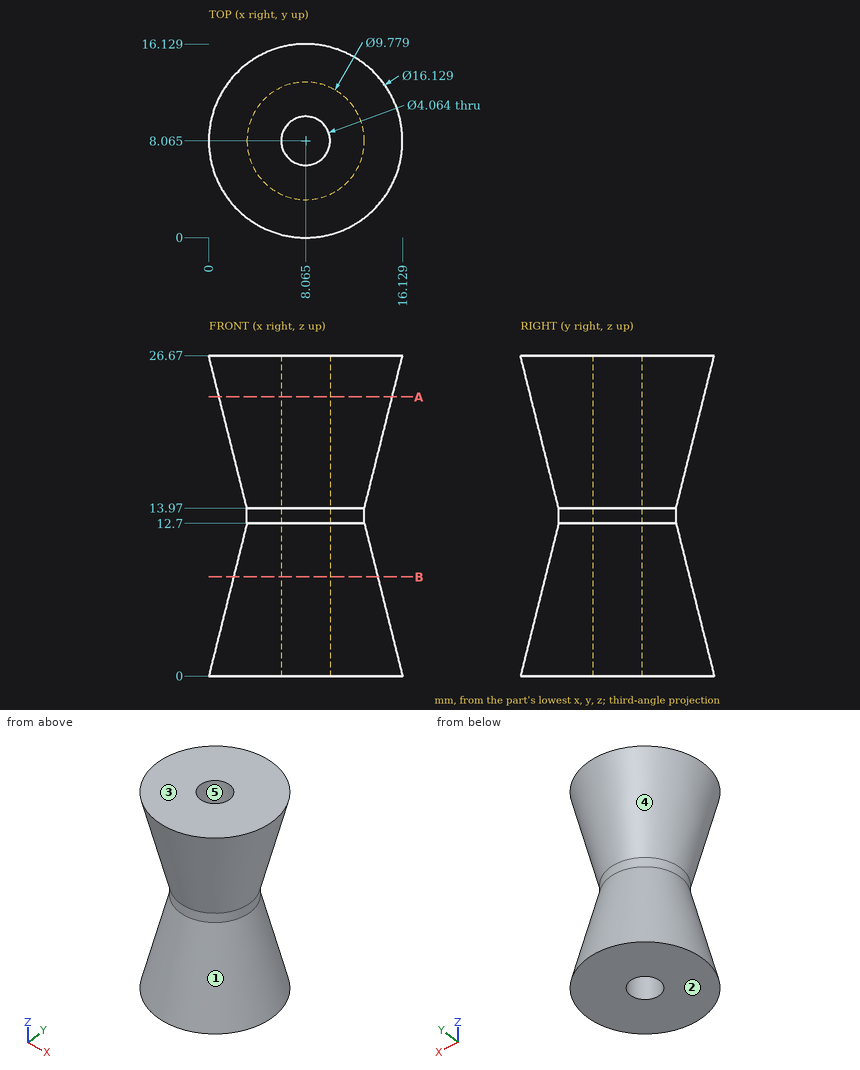
Here's the drawing with two shaded views (mm, measured from the low corner). I have some questions. A direction names the side the tool comes from. Round coordinates to 2 decimals unless told otherwise and drop trailing zeros. Loops run counter-clockwise (first coordinate to the right, second up) from the corner with the lowest first, then second, coordinate; pieces in that order, holes last.
1. Suppose I cut it at A-A, the plane z = 23.25. Please give me the cut outline in (x, y) (1 decimal), and give its area (3 significant figures).
Answers:
outline: circle Ø14.4 at (8.1, 8.1); hole circle Ø4.1 at (8.1, 8.1)
area: 150 mm2
2. Will these pins go through, and if not, where does the flat tip stop? pin 1 (4 mm diameter, centred on x = 14, z = 21, fed in from -Y); pin 2 (8 mm diameter, centred on y = 3.5, z = 20, fed in from -X) (1 decimal); pin 3 (8 mm diameter, centred on x = 6.5, z = 22, fed in from +Y).
Answers:
pin 1: stops at y = 2.58
pin 2: stops at x = 1.2
pin 3: stops at y = 15.91
3. If I drill on probe 1 along X at (y, z) = (8, 10.75) (1 decimal); probe 2 along Y at (x, z) = (8.5, 1.5); probe 3 along Y at (x, z) = (6.5, 12.25) (1 decimal), over which ranges is the centre line in solid material (lowest first)?
Answers:
probe 1: x = 2.7 to 6, 10.1 to 13.4
probe 2: y = 0.39 to 6.08, 10.05 to 15.74
probe 3: y = 3.3 to 6.8, 9.4 to 12.8
4. Thinking about a two-plate mould opening in Y: for the marked faces 3, 4 and 5, which applies, released by +Y, released by -Y, zero draft, split by the parting line, or undercut?
Answers:
face 3: zero draft
face 4: split by the parting line
face 5: undercut
5. Suppose I cut it at B-B, the plane z = 8.25. Please give me the cut outline in (x, y) (1 decimal), and give its area (3 significant figures).
Answers:
outline: circle Ø12 at (8.1, 8.1); hole circle Ø4.1 at (8.1, 8.1)
area: 100 mm2
6. For the marked faces 1 and 2, which set-ups out of +Z, -Z, +X, -X, +Y, -Y let a thin tool reach every point of the face, with its end or its side?
Answers:
face 1: none
face 2: -Z, +X, -X, +Y, -Y
